```python
from build123d import *

# Parameters (mm, degrees)
BOSS_EXTRUDE1_DEPTH = 52
BOSS_EXTRUDE2_DEPTH = 22
SKETCH1_6_R         = 9
BOSS_EXTRUDE3_DEPTH = 34
FILLET1_R           = 15


with BuildPart() as part:
    # Sketch1 → Boss-Extrude1 (new body)
    with BuildSketch(Plane.XY):
        with BuildLine():
            Line((0, 34), (108, 34))
            ThreePointArc((108, 34), (142, 0), (108, -34))
            Line((108, -34), (0, -34))
            ThreePointArc((0, -34), (-34, 0), (0, 34))
        make_face()
        with BuildLine():
            ThreePointArc((108, -15), (123, 0), (108, 15))
            Line((108, 15), (0, 15))
            ThreePointArc((0, 15), (-15, 0), (0, -15))
            Line((0, -15), (108, -15))
        make_face(mode=Mode.SUBTRACT)
    extrude(amount=BOSS_EXTRUDE1_DEPTH)

    # Sketch1_5 → Boss-Extrude2 (add)
    with BuildSketch(Plane.XY):
        with BuildLine():
            ThreePointArc((-17.626329898, 29.074258276), (-9.150825608, 32.745417858), (0, 34))
            Line((0, 34), (83, 34))
            Line((83, 34), (83, 76))
            ThreePointArc((83, 76), (86.216825102, 88.26757072), (95.03946331, 97.378131086))
            Line((95.03946331, 97.378131086), (-17.626329898, 29.074258276))
        make_face()
    extrude(amount=BOSS_EXTRUDE2_DEPTH)

    # Sketch1_6 → Boss-Extrude3 (add)
    with BuildSketch(Plane.XY):
        with BuildLine():
            Line((83, 76), (83, 34))
            Line((83, 34), (108, 34))
            ThreePointArc((108, 34), (121.647767834, 31.140623519), (133, 23.043437244))
            Line((133, 23.043437244), (133, 76))
            ThreePointArc((133, 76), (120.26757072, 97.783174898), (95.03946331, 97.378131086))
            ThreePointArc((95.03946331, 97.378131086), (86.216825102, 88.26757072), (83, 76))
        make_face()
        with Locations((108, 76)):
            Circle(SKETCH1_6_R, mode=Mode.SUBTRACT)
    extrude(amount=BOSS_EXTRUDE3_DEPTH)

    # Fillet1
    fillet1_edges = [part.edges().sort_by_distance(p)[0] for p in [
        (83, 34, 28),
    ]]
    fillet(fillet1_edges, radius=FILLET1_R)


solid = part.part
```
Could you check a few things on this model? Use its own coordinates, in mm. A direction names the side the tool comes from. Give positions to 0.01 mm unless a question says otherwise; leave off trailing zeros. Loops run counter-clockwise (first coordinate to the right, second up) from the corner with the lowest first, then second, coordinate; pieces in that order, holes last. Notation, with made-up numbers: (88, 47.5) - (125, 47.5) arc R23 ccw to (125, 59.5) - close; hole circle Ø1 at (77.5, 1.5). An arc over 180 degrees is marked (long way). Use one line per item in the form item = value.
1. I need wall thicknesses on probe 1 along Y at (x, z) = (108, 9); probe 2 along Y at (x, z) = (84, 38.5); probe 3 along Z at (x, y) = (79, 64.5). Which ranges of each line are inside material? Lowest first, please.
Response values:
probe_1 = -34 to -15, 15 to 67, 85 to 101
probe_2 = -34 to -15, 15 to 34
probe_3 = 0 to 22
2. Thinking about a two-plate mould opening in X: for faces 4 (the face through (78.72, 38.51, 28.08)), 5 (the face through (55, 15, 26)), 6 (the face through (133, 49, 17)), which applies, released by +X, released by -X, zero draft, split by the parting line, or undercut?
Response values:
face_4 = released by -X
face_5 = undercut
face_6 = released by +X
3. I want a section at A-A (z = 17). Please give me the cut outline in (x, y), and give its area (3 significant figures).
Response values:
outline = (-17.63, 29.07) arc R34 ccw to (0, -34) - (108, -34) arc R34 ccw to (133, 23.04) - (133, 76) arc R25 ccw to (95.04, 97.38) - close; hole (0, -15) - (108, -15) arc R15 ccw to (108, 15) - (0, 15) arc R15 ccw to start; hole circle Ø18 at (108, 76)
area = 12,600 mm²
4. I'm going to push flat-ended pins straight in: pin 1 Ø1 at (y, z) = (66, 19.5) entering from -X; pin 2 Ø6 at (x, y) = (74.5, 73.5) entering from +Z; pin 3 Ø6 at (y, z) = (11.5, 22.5) entering from -X. Where does each tip first touch, or does it pass through?
Response values:
pin_1 = 42.46
pin_2 = 22
pin_3 = -32.92
5. I want a section at B-B (y = 82.5). Please give me the cut outline in (x, z), and give its area (3 significant figures).
Response values:
outline = (70.5, 0) - (101.78, 0) - (101.78, 34) - (83.86, 34) - (83.86, 22) - (70.5, 22) - close; (114.22, 0) - (132.14, 0) - (132.14, 34) - (114.22, 34) - close
area = 1,510 mm²
6. On a 3-axis mill with a long thin cutter (end or side, diameter ignored), from which of +Z, -Z, +X, -X, +Y, -Y can I reach the whole of each face in a straight line? I mean faces 1 (the face through (-15, 0, 26)), 2 (the face through (41, 34, 37)), 3 (the face through (72, 34, 0)). Say none if no direction works.
Response values:
face_1 = +Z, -Z
face_2 = +Z, -X, +Y
face_3 = -Z, +X, -X, +Y, -Y
7. I want a section at C-C (x = 119). Please give me the cut outline in (y, z).
Response values:
outline = (-32.17, 0) - (-10.2, 0) - (-10.2, 52) - (-32.17, 52) - close; (10.2, 0) - (98.45, 0) - (98.45, 34) - (32.17, 34) - (32.17, 52) - (10.2, 52) - close
8. I want a section at D-D (z = 43). Please give me the cut outline in (x, y), and give its area (3 significant figures).
Response values:
outline = (0, -34) - (108, -34) arc R34 ccw to (108, 34) - (0, 34) arc R34 ccw to start; hole (0, -15) - (108, -15) arc R15 ccw to (108, 15) - (0, 15) arc R15 ccw to start
area = 7,030 mm²
